Geometry: final body of the model. Coordinates: model frame, mm. Round coordinates to 2 decimals unless told otherwise and drop trailing zeros. Loops run counter-clockwise (first coordinate to the right, second up) from the corner with the lowest first, then second, coordinate; pieces in that order, holes last. Notation, with made-up numbers: (29.5, 22.5) -> (40.5, 22.5) arc R22 ccw to (40.5, 47.5) -> close; hole circle Ø4 at (-27, 82). An arc over 180 degrees is marked (long way). Answer in a Markdown table with one row per item.
```python
from build123d import *

# Parameters (mm, degrees)
CROQUIS1_R              = 35
CROQUIS1_R_2            = 1.5
CROQUIS1_R_3            = 29
SALIENTE_EXTRUIR3_DEPTH = 14.1
CROQUIS4_R              = 29
CROQUIS4_R_2            = 25
SALIENTE_EXTRUIR4_DEPTH = 14.1
CROQUIS5_R              = 29
CORTAR_EXTRUIR1_DEPTH   = 1.1
CORTAR_EXTRUIR1_DRAFT   = -76
SALIENTE_EXTRUIR5_START = -3.1
CROQUIS6_R              = 29
CROQUIS6_R_2            = 25
SALIENTE_EXTRUIR5_DEPTH = 3.1
CROQUIS7_R              = 29
CROQUIS7_R_2            = 27
CORTAR_EXTRUIR2_DEPTH   = 1
CROQUIS11_R             = 1
CORTAR_EXTRUIR5_DEPTH   = 4


with BuildPart() as part:
    # Croquis1 → Saliente-Extruir3 (new body)
    with BuildSketch(Plane.XY):
        Circle(CROQUIS1_R)
        with Locations((0, 32)):
            Circle(CROQUIS1_R_2, mode=Mode.SUBTRACT)
        with Locations((22.627416998, 22.627416998)):
            Circle(CROQUIS1_R_2, mode=Mode.SUBTRACT)
        with Locations((32, 0)):
            Circle(CROQUIS1_R_2, mode=Mode.SUBTRACT)
        with Locations((22.627416998, -22.627416998)):
            Circle(CROQUIS1_R_2, mode=Mode.SUBTRACT)
        with Locations((0, -32)):
            Circle(CROQUIS1_R_2, mode=Mode.SUBTRACT)
        with Locations((-22.627416998, -22.627416998)):
            Circle(CROQUIS1_R_2, mode=Mode.SUBTRACT)
        with Locations((-32, 0)):
            Circle(CROQUIS1_R_2, mode=Mode.SUBTRACT)
        with Locations((-22.627416998, 22.627416998)):
            Circle(CROQUIS1_R_2, mode=Mode.SUBTRACT)
        Circle(CROQUIS1_R_3, mode=Mode.SUBTRACT)
    extrude(amount=SALIENTE_EXTRUIR3_DEPTH)



with BuildPart() as body_2:
    # Croquis4 → Saliente-Extruir4 (new body)
    with BuildSketch(Plane(origin=(0, 0, 0), x_dir=(-1, 0, 0), z_dir=(0, 0, -1))):
        with Locations(Location((0, 0, 0), (0, 0, 180))):
            Circle(CROQUIS4_R)
        Circle(CROQUIS4_R_2, mode=Mode.SUBTRACT)
    extrude(amount=-SALIENTE_EXTRUIR4_DEPTH)


with BuildPart() as cortar_extruir1_tool:
    # Croquis5 → Cortar-Extruir1 (with draft: the straight prism first)
    with BuildSketch(Plane(origin=(0, 0, 0), x_dir=(-1, 0, 0), z_dir=(0, 0, -1))):
        with Locations(Location((0, 0, 0), (0, 0, 180))):
            Circle(CROQUIS5_R)
    extrude(amount=-CORTAR_EXTRUIR1_DEPTH)
    # Cortar-Extruir1: the draft: its side faces are tilted about the plane it starts from
    cortar_extruir1_sides = [cortar_extruir1_tool.faces().sort_by_distance(p)[0] for p in [
        (-29, 0, 0.55),
    ]]
    draft(cortar_extruir1_sides, Plane(origin=(0, 0, 0), x_dir=(-1, 0, 0), z_dir=(0, 0, -1)), CORTAR_EXTRUIR1_DRAFT)


with BuildPart() as body_2_1:
    add(body_2.part)

    # Cortar-Extruir1: cut by cortar_extruir1_tool
    add(cortar_extruir1_tool.part, mode=Mode.SUBTRACT)


with BuildPart() as part_1:
    add(part.part)

    add(body_2_1.part)  # Saliente-Extruir5 merges body 2
    # Croquis6 → Saliente-Extruir5 (add)
    with BuildSketch(Plane.XY.offset(14.1).offset(SALIENTE_EXTRUIR5_START)):
        Circle(CROQUIS6_R)
        Circle(CROQUIS6_R_2, mode=Mode.SUBTRACT)
    extrude(amount=SALIENTE_EXTRUIR5_DEPTH)

    # Croquis7 → Cortar-Extruir2 (cut)
    with BuildSketch(Plane.XY.offset(14.1)):
        Circle(CROQUIS7_R)
        Circle(CROQUIS7_R_2, mode=Mode.SUBTRACT)
    extrude(amount=-CORTAR_EXTRUIR2_DEPTH, mode=Mode.SUBTRACT)

    # Cortar-Extruir3 cone 1 section (through the dimple's axis) → Cortar-Extruir3 (revolve, cut)
    with BuildSketch(Plane(origin=(0, 32, 0), x_dir=(0, 1, 0), z_dir=(1, 0, 0))):
        Polygon((0, 0), (1.7, 0), (0, 0.299755867), align=None)
    revolve(axis=Axis((0, 32, 0), (0, 0, 1)), mode=Mode.SUBTRACT)

    # Cortar-Extruir3 cone 2 section (through the dimple's axis) → Cortar-Extruir3 cone 2 (revolve, cut)
    with BuildSketch(Plane(origin=(-22.627416998, 22.627416998, 0), x_dir=(0, 1, 0), z_dir=(1, 0, 0))):
        Polygon((0, 0), (1.7, 0), (0, 0.299755867), align=None)
    revolve(axis=Axis((-22.627416998, 22.627416998, 0), (0, 0, 1)), mode=Mode.SUBTRACT)

    # Cortar-Extruir3 cone 3 section (through the dimple's axis) → Cortar-Extruir3 cone 3 (revolve, cut)
    with BuildSketch(Plane.YZ.offset(-32)):
        Polygon((0, 0), (1.7, 0), (0, 0.299755867), align=None)
    revolve(axis=Axis((-32, 0, 0), (0, 0, 1)), mode=Mode.SUBTRACT)

    # Cortar-Extruir3 cone 4 section (through the dimple's axis) → Cortar-Extruir3 cone 4 (revolve, cut)
    with BuildSketch(Plane(origin=(-22.627416998, -22.627416998, 0), x_dir=(0, 1, 0), z_dir=(1, 0, 0))):
        Polygon((0, 0), (1.7, 0), (0, 0.299755867), align=None)
    revolve(axis=Axis((-22.627416998, -22.627416998, 0), (0, 0, 1)), mode=Mode.SUBTRACT)

    # Cortar-Extruir3 cone 5 section (through the dimple's axis) → Cortar-Extruir3 cone 5 (revolve, cut)
    with BuildSketch(Plane(origin=(0, -32, 0), x_dir=(0, 1, 0), z_dir=(1, 0, 0))):
        Polygon((0, 0), (1.7, 0), (0, 0.299755867), align=None)
    revolve(axis=Axis((0, -32, 0), (0, 0, 1)), mode=Mode.SUBTRACT)

    # Cortar-Extruir3 cone 6 section (through the dimple's axis) → Cortar-Extruir3 cone 6 (revolve, cut)
    with BuildSketch(Plane(origin=(22.627416998, -22.627416998, 0), x_dir=(0, 1, 0), z_dir=(1, 0, 0))):
        Polygon((0, 0), (1.7, 0), (0, 0.299755867), align=None)
    revolve(axis=Axis((22.627416998, -22.627416998, 0), (0, 0, 1)), mode=Mode.SUBTRACT)

    # Cortar-Extruir3 cone 7 section (through the dimple's axis) → Cortar-Extruir3 cone 7 (revolve, cut)
    with BuildSketch(Plane.YZ.offset(32)):
        Polygon((0, 0), (1.7, 0), (0, 0.299755867), align=None)
    revolve(axis=Axis((32, 0, 0), (0, 0, 1)), mode=Mode.SUBTRACT)

    # Cortar-Extruir3 cone 8 section (through the dimple's axis) → Cortar-Extruir3 cone 8 (revolve, cut)
    with BuildSketch(Plane(origin=(22.627416998, 22.627416998, 0), x_dir=(0, 1, 0), z_dir=(1, 0, 0))):
        Polygon((0, 0), (1.7, 0), (0, 0.299755867), align=None)
    revolve(axis=Axis((22.627416998, 22.627416998, 0), (0, 0, 1)), mode=Mode.SUBTRACT)

    # Cortar-Extruir4 cone 1 section (through the dimple's axis) → Cortar-Extruir4 (revolve, cut)
    with BuildSketch(Plane(origin=(0, 32, 14.1), x_dir=(0, -1, 0), z_dir=(1, 0, 0))):
        Polygon((0, 0), (1.7, 0), (0, 0.299755867), align=None)
    revolve(axis=Axis((0, 32, 14.1), (0, 0, -1)), mode=Mode.SUBTRACT)

    # Cortar-Extruir4 cone 2 section (through the dimple's axis) → Cortar-Extruir4 cone 2 (revolve, cut)
    with BuildSketch(Plane(origin=(22.627416998, 22.627416998, 14.1), x_dir=(0, -1, 0), z_dir=(1, 0, 0))):
        Polygon((0, 0), (1.7, 0), (0, 0.299755867), align=None)
    revolve(axis=Axis((22.627416998, 22.627416998, 14.1), (0, 0, -1)), mode=Mode.SUBTRACT)

    # Cortar-Extruir4 cone 3 section (through the dimple's axis) → Cortar-Extruir4 cone 3 (revolve, cut)
    with BuildSketch(Plane(origin=(32, 0, 14.1), x_dir=(0, -1, 0), z_dir=(1, 0, 0))):
        Polygon((0, 0), (1.7, 0), (0, 0.299755867), align=None)
    revolve(axis=Axis((32, 0, 14.1), (0, 0, -1)), mode=Mode.SUBTRACT)

    # Cortar-Extruir4 cone 4 section (through the dimple's axis) → Cortar-Extruir4 cone 4 (revolve, cut)
    with BuildSketch(Plane(origin=(22.627416998, -22.627416998, 14.1), x_dir=(0, -1, 0), z_dir=(1, 0, 0))):
        Polygon((0, 0), (1.7, 0), (0, 0.299755867), align=None)
    revolve(axis=Axis((22.627416998, -22.627416998, 14.1), (0, 0, -1)), mode=Mode.SUBTRACT)

    # Cortar-Extruir4 cone 5 section (through the dimple's axis) → Cortar-Extruir4 cone 5 (revolve, cut)
    with BuildSketch(Plane(origin=(0, -32, 14.1), x_dir=(0, -1, 0), z_dir=(1, 0, 0))):
        Polygon((0, 0), (1.7, 0), (0, 0.299755867), align=None)
    revolve(axis=Axis((0, -32, 14.1), (0, 0, -1)), mode=Mode.SUBTRACT)

    # Cortar-Extruir4 cone 6 section (through the dimple's axis) → Cortar-Extruir4 cone 6 (revolve, cut)
    with BuildSketch(Plane(origin=(-22.627416998, -22.627416998, 14.1), x_dir=(0, -1, 0), z_dir=(1, 0, 0))):
        Polygon((0, 0), (1.7, 0), (0, 0.299755867), align=None)
    revolve(axis=Axis((-22.627416998, -22.627416998, 14.1), (0, 0, -1)), mode=Mode.SUBTRACT)

    # Cortar-Extruir4 cone 7 section (through the dimple's axis) → Cortar-Extruir4 cone 7 (revolve, cut)
    with BuildSketch(Plane(origin=(-32, 0, 14.1), x_dir=(0, -1, 0), z_dir=(1, 0, 0))):
        Polygon((0, 0), (1.7, 0), (0, 0.299755867), align=None)
    revolve(axis=Axis((-32, 0, 14.1), (0, 0, -1)), mode=Mode.SUBTRACT)

    # Cortar-Extruir4 cone 8 section (through the dimple's axis) → Cortar-Extruir4 cone 8 (revolve, cut)
    with BuildSketch(Plane(origin=(-22.627416998, 22.627416998, 14.1), x_dir=(0, -1, 0), z_dir=(1, 0, 0))):
        Polygon((0, 0), (1.7, 0), (0, 0.299755867), align=None)
    revolve(axis=Axis((-22.627416998, 22.627416998, 14.1), (0, 0, -1)), mode=Mode.SUBTRACT)

    # Croquis11 → Cortar-Extruir5 (cut)
    with BuildSketch(Plane.XY.offset(14.1)):
        with Locations((29.56414504, 12.245869836)):
            Circle(CROQUIS11_R)
        with Locations((-29.56414504, -12.245869836)):
            Circle(CROQUIS11_R)
    extrude(amount=-CORTAR_EXTRUIR5_DEPTH, mode=Mode.SUBTRACT)

    # Cortar-Extruir6 cone 1 section (through the dimple's axis) → Cortar-Extruir6 (revolve, cut)
    with BuildSketch(Plane(origin=(29.56414504, 12.245869836, 14.1), x_dir=(0, -1, 0), z_dir=(1, 0, 0))):
        Polygon((0, 0), (1.2, 0), (0, 0.211592377), align=None)
    revolve(axis=Axis((29.56414504, 12.245869836, 14.1), (0, 0, -1)), mode=Mode.SUBTRACT)

    # Cortar-Extruir6 cone 2 section (through the dimple's axis) → Cortar-Extruir6 cone 2 (revolve, cut)
    with BuildSketch(Plane(origin=(-29.56414504, -12.245869836, 14.1), x_dir=(0, -1, 0), z_dir=(1, 0, 0))):
        Polygon((0, 0), (1.2, 0), (0, 0.211592377), align=None)
    revolve(axis=Axis((-29.56414504, -12.245869836, 14.1), (0, 0, -1)), mode=Mode.SUBTRACT)


solid = part_1.part
```
Item 1: Cut plane A-A (x = 0). Count the separate pieces of the cut face and the enclosed holes in it, then the cut area to 3 significant figures.
Answer:
| item | result |
|---|---|
| separate pieces | 4 |
| enclosed holes | 0 |
| area | 189 mm² |
Item 2: Pin query (flat end, axial travel): pin 1 Ø1.6 at (x, y) = (-29.5, -12) entering from +Z; pin 2 Ø2.5 at (x, y) = (22.63, 22.63) entering from -Z; pin 3 Ø4 at (y, z) = (-2.5, 12) entering from +X; pin 4 Ø2 at (y, z) = (-8.5, 9) entering from +X. Return the tip coordinate at first contact, or that it passes through.
Answer:
| item | result |
|---|---|
| pin 1 | stops at z = 14.07 |
| pin 2 | passes through |
| pin 3 | stops at x = 35 |
| pin 4 | stops at x = 34.19 |
Item 3: Cut plane B-B (x = 32). Output: boundary loops of the cut face in (y, z).
Answer:
| item | result |
|---|---|
| outline | (-14.18, 0) -> (-1.7, 0) -> (-1.5, 0.04) -> (-1.5, 14.06) -> (-1.7, 14.1) -> (-14.18, 14.1) -> close; (1.5, 0.04) -> (1.7, 0) -> (14.18, 0) -> (14.18, 14.1) -> (1.7, 14.1) -> (1.5, 14.06) -> close |
Item 4: Draft query along Y for faces 1 (the face through (30.5, 0.07, 6.95)), 2 (the face through (8, -26, 13.1)), 3 (the face through (-28, -21, 7)), 4 (the face through (-21, 21, 0)). Return one class per face: pulls with the +Y half, pulls with the -Y half, needs draft (parallel to the pull), parting line crosses it, or undercut.
Answer:
| item | result |
|---|---|
| face 1 | undercut |
| face 2 | undercut |
| face 3 | parting line crosses it |
| face 4 | needs draft |
Item 5: Line query: probe 1 along Y at (x, z) = (0, 5); probe 2 along Y at (x, z) = (0, 13.45); probe 3 along Y at (x, z) = (-16.5, 13.25). Output: solid intervals per line, ascending. Write a range as [from, to].
Answer:
| item | result |
|---|---|
| probe 1 | y = [-35, -33.5], [-30.5, -25], [25, 30.5], [33.5, 35] |
| probe 2 | y = [-35, -33.5], [-30.5, -29], [-27, -25], [25, 27], [29, 30.5], [33.5, 35] |
| probe 3 | y = [-30.87, -23.85], [-21.37, -18.78], [18.78, 21.37], [23.85, 30.87] |
